```python
from build123d import *

# Parameters (mm, degrees)
SKETCH2_R           = 47.5
SKETCH2_R_2         = 40
BOSS_EXTRUDE2_DEPTH = 7.5
CIRPATTERN1_COUNT   = 12


with BuildPart() as part:
    # Sketch2 → Boss-Extrude2 (new body)
    with BuildSketch(Plane(origin=(0, 0, 0), x_dir=(1, 0, 0), z_dir=(0, 1, 0))):
        with Locations(Location((0, 0, 0), (0, 0, 270))):
            Circle(SKETCH2_R)
        with Locations(Location((0, 0, 0), (0, 0, 270))):
            Circle(SKETCH2_R_2, mode=Mode.SUBTRACT)
    extrude(amount=-BOSS_EXTRUDE2_DEPTH)

    # Loft2: read off the stored shape, not the designer's step
    # Loft2: loft between two sections, ruled curve by curve
    loft2_from = [
        Edge.make_bspline([(-5.700542846, 0, -47.156694236), (-5.750547608, 0, -47.570349449), (-5.80055237, 0, -47.984004661), (-5.900561893, 0, -48.811315086), (-5.950566655, 0, -49.224970299), (-6.000571417, 0, -49.638625511)], [0, 0, 0, 0, 0.5, 0.5, 1, 1, 1, 1], 3),
        Edge.make_bspline([(-6.000571417, 0, -49.638625511), (-3.977812454, 0, -49.88314698), (-1.943898665, 0, -50.003725887), (0.093582631, 0, -49.999912423)], [0, 0, 0, 0, 1, 1, 1, 1], 3, [1, 0.998756532, 0.998756532, 1]),
        Edge.make_bspline([(0.093582631, 0, -49.999912423), (0.092802776, 0, -49.583246486), (0.092022921, 0, -49.166580549), (0.09046321, 0, -48.333248675), (0.089683355, 0, -47.916582739), (0.088903499, 0, -47.499916802)], [0, 0, 0, 0, 0.5, 0.5, 1, 1, 1, 1], 3),
        Edge.make_line((0.088903499, 0, -47.499916802), (-5.700542846, 0, -47.156694236)),
    ]
    loft2_to = [
        Edge.make_bspline([(0.088903499, -7.5, -47.499916802), (0.089683355, -7.5, -47.916582739), (0.09046321, -7.5, -48.333248675), (0.092022921, -7.5, -49.166580549), (0.092802776, -7.5, -49.583246486), (0.093582631, -7.5, -49.999912423)], [0, 0, 0, 0, 0.5, 0.5, 1, 1, 1, 1], 3),
        Edge.make_bspline([(0.093582631, -7.5, -49.999912423), (2.131063927, -7.5, -49.996098959), (4.164512103, -7.5, -49.867907351), (6.186341578, -7.5, -49.615815804)], [0, 0, 0, 0, 1, 1, 1, 1], 3, [1, 0.998756532, 0.998756532, 1]),
        Edge.make_bspline([(6.186341578, -7.5, -49.615815804), (6.134788731, -7.5, -49.202350672), (6.083235885, -7.5, -48.78888554), (5.980130192, -7.5, -47.961955277), (5.928577345, -7.5, -47.548490145), (5.877024499, -7.5, -47.135025014)], [0, 0, 0, 0, 0.5, 0.5, 1, 1, 1, 1], 3),
        Edge.make_line((5.877024499, -7.5, -47.135025014), (0.088903499, -7.5, -47.499916802)),
    ]
    loft2 = Solid(Shell([*[Face.make_surface_from_curves(loft2_from[k], loft2_to[k]) for k in range(4)], Face(Wire(loft2_from)), Face(Wire(loft2_to))]))
    add(loft2)

    # CirPattern1: Loft2 ×12 about axis
    cirpattern1_axis = Axis((0, 0, 0), (0, 1, 0))
    for i in range(1, CIRPATTERN1_COUNT):
        add(loft2.rotate(cirpattern1_axis, i * 360 / CIRPATTERN1_COUNT))


solid = part.part
```
The listing builds one solid part. Answer for the finished solid, in the listing's coordinates (mm). Coordinates: 2 decimals unless noted, no trailing zeros. Order: outer loops, then holes, each group sorted by start corner. A loop starts at its lowest first (then second) coordinate and runs counter-clockwise, first axis right, second up. Notation, with made-up numbers: M 6,11.5 L 41,11.5 A8 ccw 41,15.5 Z; hole C 34.25,2.25 d4. An arc over 180 degrees is marked long. Answer as a JSON object with one key per item and string values. Group by question number.
1. Section A-A on z = -36 is taken. Write down the section's boundary in (x, y), then the cut area to 3 significant figures.
2. Flat-ended cylindrical pins translate along their axes: P1, Ø2, axis at y = -1.5, z = -18, coming from the +X side; P2, Ø2, axis at x = 32.5, y = -2.5, coming from the -Z side. Find the tip coordinate at first contact, or state that the pin passes through.
3. Straight lines are drawn through the part: line 1 (Z direction, x = -43.5, y = -4.5); line 2 (X direction, y = -4.75, z = 0); line 3 (Z direction, x = -44, y = -4.25). For each, find the intervals that lie inside material, in ascending order.
4. Section B-B on z = -9.5 is taken. Write down the section's boundary in (x, y).
Values follow:
{
 "1": {"outline": "M -30.99,-7.5 L -17.44,-7.5 L -17.44,0 L -30.99,0 Z; M 17.44,-7.5 L 30.99,-7.5 L 30.99,0 L 17.44,0 Z", "area": "203 mm2"},
 "2": {"P1": "x = 44.35", "P2": "z = -35.55"},
 "3": {"line 1": "-24.47 to -22.46, -19.08 to 19.08, 20.93 to 24.47", "line 2": "-49.91 to -40, 40 to 49.91", "line 3": "-23.56 to -22.49, -17.9 to 17.9, 21.39 to 23.56"},
 "4": {"outline": "M -46.54,-7.5 L -38.86,-7.5 L -38.86,0 L -46.54,0 Z; M 38.86,-7.5 L 46.54,-7.5 L 46.54,0 L 38.86,0 Z"}
}
